from build123d import *

# Parameters (mm, degrees)
F1_DEPTH = 3.175
F2_R     = 5
F3_R     = 30
F5_DEPTH = 1.5875


with BuildPart() as f1:
    # F0 (on Front) → F1 (new body)
    with BuildSketch(Plane.XZ):
        with BuildLine():
            Line((-75, 103.6675041929), (-75, 0))
            Line((-75, 0), (75, 0))
            Line((75, 0), (75, 103.6675041929))
            ThreePointArc((75, 103.6675041929), (64.2261628933, 142.397337655), (35, 170))
            Line((35, 170), (49.8954840004, 204.6374976635))
            Line((49.8954840004, 204.6374976635), (37.5165957212, 290))
            Line((37.5165957212, 290), (-42.4834042788, 290))
            ThreePointArc((-42.4834042788, 290), (-44.7601701514, 229.6246780894), (-35, 170))
            ThreePointArc((-35, 170), (-64.2261628933, 142.397337655), (-75, 103.6675041929))
        make_face()
    extrude(amount=F1_DEPTH)

    # F2
    f2_edges = [f1.edges().sort_by_distance(p)[0] for p in [
        (-35, -1.5875, 170),
        (-42.483404, -1.5875, 290),
        (37.516596, -1.5875, 290),
        (75, -1.5875, 0),
        (-75, -1.5875, 0),
        (35, -1.5875, 170),
    ]]
    fillet(f2_edges, radius=F2_R)

    # F3
    f3_edges = [f1.edges().sort_by_distance(p)[0] for p in [
        (49.895484, -1.5875, 204.637498),
    ]]
    fillet(f3_edges, radius=F3_R)

    # F4 (on face) → F5 (cut)
    with BuildSketch(Plane.XZ.offset(3.175)):
        with BuildLine():
            Line((33.1893731308, 290), (-31.6550214826, 290))
            Line((-31.6550214826, 290), (-31.6550214826, 245))
            Line((-31.6550214826, 245), (29.5949785174, 245))
            Line((29.5949785174, 245), (41.1419839012, 265))
            Line((41.1419839012, 265), (38.137614304, 285.7175718024))
            ThreePointArc((38.137614304, 285.7175718024), (36.461386348, 288.7807313454), (33.1893731308, 290))
        make_face()
    extrude(amount=-F5_DEPTH, mode=Mode.SUBTRACT)


solid = f1.part
Source: CAD feature listing. Evaluate the final solid. Frame: model axes, mm. A direction names the side the tool comes from. Coordinates: 2 decimals unless noted, no trailing zeros. Loops run counter-clockwise (first coordinate to the right, second up) from the corner with the lowest first, then second, coordinate; pieces in that order, holes last. Notation, with made-up numbers: (72.25, 17) - (98.25, 17) arc R32 ccw to (98.25, 44) - close; hole circle Ø10 at (14.25, 35.5). An arc over 180 degrees is marked (long way). Return JSON: item names as keys, results as strings.
Q1. Section A-A, the plane x = -11. Return loops of the section in (y, z) (1 decimal).
Results:
{"outline": "(-3.2, 0) - (0, 0) - (0, 290) - (-1.6, 290) - (-1.6, 245) - (-3.2, 245) - close"}
Q2. Material intervals for line 1 along Z through (x, y) = (29, -2.9); line 2 along X through (y, z) = (-1.75, 246.5); line 3 along X through (y, z) = (-0.75, 115), sorted ascending.
Results:
{"line 1": "0 to 245", "line 2": "-45.34 to -31.66, 30.46 to 43.82", "line 3": "-74.14 to 74.14"}
Q3. Access query for faces 1 (the flat face through (35.288, -2.392, 254.86)), 2 (the flat face through (41.592, -1.565, 185.33)), 3 (the flat face through (-1, 0, 115)). Directions: +Z, -Z, +X, -X, +Y, -Y. A direction counts if a zero-diameter tool reaches every point of the face in a straight line with its end or side. Return the directions, or none.
Results:
{"face 1": "+Z, -Y", "face 2": "+X, +Y, -Y", "face 3": "+Z, -Z, +X, -X, +Y"}
Q4. Mould query, pull axis Z, two halves, no side actions, for faces 4 (the cylindrical face through (-44.79, -1.57, 230.12)), 5 (the cylindrical face through (-74, -2, 2)), 6 (the flat face through (4, -1.588, 268)). Classes: released by +Z, released by -Z, zero draft, split by the parting line, or undercut.
Results:
{"face 4": "undercut", "face 5": "released by -Z", "face 6": "zero draft"}
Q5. Contact query for flat-ended pins moving along their axis: P1, Ø1.7, axis at x = 7, y = -2.5, coming from the +Z side; P2, Ø13.5, axis at x = 21, z = 257.5, coming from the -Y side; P3, Ø1.3, axis at y = -2.5, z = 276, coming from the +X side (3 decimals). Output: stop coordinate, or through.
Results:
{"P1": "z = 245", "P2": "y = -1.59", "P3": "x = -31.655"}
Q6. Section C-C, the plane z = 149. Return loops of the section in (x, y) (3 decimals), plus the area to 3 significant figures.
Results:
{"outline": "(-59.749, -3.175) - (59.749, -3.175) - (59.749, 0) - (-59.749, 0) - close", "area": "379 mm2"}
Q7. Section B-B, the plane z = 208.5. Return loops of the section in (x, y) (3 decimals).
Results:
{"outline": "(-42.697, -3.175) - (48.99, -3.175) - (48.99, 0) - (-42.697, 0) - close"}
